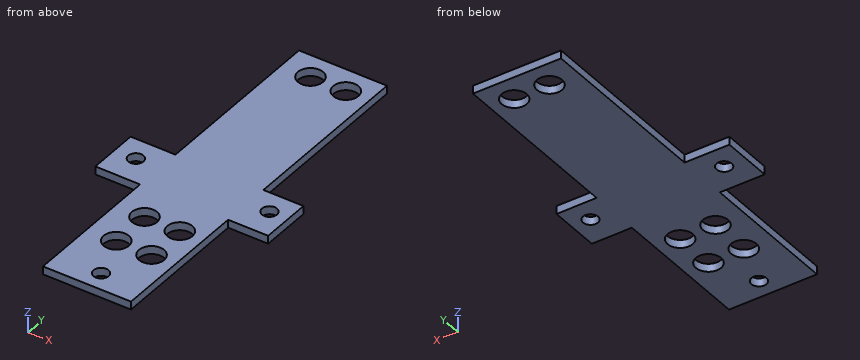
Autodesk Inventor part; units mm, degrees
ref_plane "YZ Plane" through (0, 0, 0) normal (1, 0, 0) x (0, 1, 0)
ref_plane "XZ Plane" through (0, 0, 0) normal (0, 1, 0) x (-1, 0, 0)
ref_plane "XY Plane" through (0, 0, 0) normal (0, 0, 1) x (1, 0, 0)
sketch "Эскиз1" plane through (0, 0, 0) normal (0, 0, 1) x (1, 0, 0)
  line L0 (0, -8.89) -> (17.45, -8.89)
  line L1 (17.45, -8.89) -> (17.453, 19.05)
  line L2 (17.453, 19.05) -> (25.4, 19.05)
  line L3 (25.4, 19.05) -> (25.4, 29.21)
  line L4 (25.4, 29.21) -> (17.45, 29.21)
  line L5 (17.45, 29.21) -> (17.45, 64.76)
  line L6 (17.45, 64.76) -> (0, 64.76)
  line L7 (0, 64.76) -> (0, 29.21)
  line L8 (0, 29.21) -> (-8.89, 29.21)
  line L9 (-8.89, 29.21) -> (-8.89, 19.05)
  line L10 (-8.89, 19.05) -> (0, 19.05)
  line L11 (0, 19.05) -> (0, -8.89)
  circle A0 centre (5.77, 3.81) radius 2.5
  circle A1 centre (12.77, 3.81) radius 2.5
  circle A2 centre (5.77, 11.94) radius 2.5
  circle A3 centre (12.77, 11.94) radius 2.5
  circle A4 centre (5.77, 59.69) radius 2.5
  circle A5 centre (12.77, 59.69) radius 2.5
  circle A6 centre (8.89, -5.08) radius 1.5
  circle A7 centre (-4.699, 24.638) radius 1.5
  circle A8 centre (21.717, 24.765) radius 1.5
extrude "xt60_pcb.brdКонтур" add sketch "Эскиз1" along normal blind 1.6
properties part number "xt60_pcb.brdКонтур"
Can you work these out from the model? Positions are in its coordinate system, mm. Coordinates: 2 decimals unless noted, no trailing zeros. Write each loop counter-clockwise with the first axis right and the second up, starting at its lowest first coordinate (ties: lowest second). Pieces come first, ordered by that corner, then holes. Notation, with made-up numbers: M 88,29.25 L 118,29.25 A21 ccw 118,41.25 Z; hole C 83.25,-33.5 d11. An arc over 180 degrees is marked long. Answer as CSV lines item,"result".
Item 1: Imagine slicing it at A-A on x = 12.77. List the corners of the cut face in (y, z) for me, plus the area to 3 significant figures.
Geometry results:
outline,"M -8.89,0 L 1.31,0 L 1.31,1.6 L -8.89,1.6 Z; M 6.31,0 L 9.44,0 L 9.44,1.6 L 6.31,1.6 Z; M 14.44,0 L 57.19,0 L 57.19,1.6 L 14.44,1.6 Z; M 62.19,0 L 64.76,0 L 64.76,1.6 L 62.19,1.6 Z"
area,"93.8 mm2"
Item 2: Imagine slicing it at D-D on y = 3.81. List the corners of the cut face in (x, z) for me.
Geometry results:
outline,"M 0,0 L 3.27,0 L 3.27,1.6 L 0,1.6 Z; M 8.27,0 L 10.27,0 L 10.27,1.6 L 8.27,1.6 Z; M 15.27,0 L 17.45,0 L 17.45,1.6 L 15.27,1.6 Z"
Item 3: I'm going to push flat-ended pins straight in: P1, Ø0.8, axis at x = 20, z = 1, coming from the +Y side; P2, Ø0.8, axis at y = 52.5, z = 0.5, coming from the +X side; P3, Ø3, axis at x = 5.77, y = 3.81, coming from the +Z side; P4, Ø0.5, axis at y = 10.5, z = 1, coming from the +X side. Where does each tip first touch, or does it pass through?
Geometry results:
P1,"stops at y = 29.21"
P2,"stops at x = 17.45"
P3,"passes through"
P4,"stops at x = 17.45"
Item 4: Imagine slicing it at C-C on x = 21. List the corners of the cut face in (y, z) for me, plus the area to 3 significant figures.
Geometry results:
outline,"M 19.05,0 L 23.45,0 L 23.45,1.6 L 19.05,1.6 Z; M 26.08,0 L 29.21,0 L 29.21,1.6 L 26.08,1.6 Z"
area,"12.0 mm2"
Item 5: Imagine slicing it at B-B on y = -5.08. List the corners of the cut face in (x, z) for me.
Geometry results:
outline,"M 0,0 L 7.39,0 L 7.39,1.6 L 0,1.6 Z; M 10.39,0 L 17.45,0 L 17.45,1.6 L 10.39,1.6 Z"
Item 6: Please list where these lines run through material, in increasing order: line 1 along Y through (x, z) = (12.77, 0.7); line 2 along X through (y, z) = (11, 1.45); line 3 along Y through (x, z) = (15, 1.05).
Geometry results:
line 1,"y = -8.89 to 1.31, 6.31 to 9.44, 14.44 to 57.19, 62.19 to 64.76"
line 2,"x = 0 to 3.45, 8.09 to 10.45, 15.09 to 17.45"
line 3,"y = -8.89 to 2.68, 4.94 to 10.81, 13.07 to 58.56, 60.82 to 64.76"
